Build history of the part. All positions in model axes, mm. A direction names the side the tool comes from. Round coordinates to 2 decimals unless told otherwise and drop trailing zeros. Write each loop counter-clockwise with the first axis right and the second up, starting at its lowest first coordinate (ties: lowest second). Pieces come first, ordered by that corner, then holes.
Item 1: Band-saw the part on A-A, the plane y = 0. Write the cut outline in (x, z), then the cut area to 3 significant figures.
Item 2: Band-saw the part on B-B, the plane x = -12.5. Write the cut outline in (y, z).
Item 3: 3-axis set-ups, long thin cutter, end or side, ignore diameter. For faces 1 (the flat face through (42, -15, 4)), 2 (the flat face through (16, -15, 8)): which of +Z, -Z, +X, -X, +Y, -Y reach the whole face in a straight line?
Item 4: Drop flat-ended pins along their axis: pin 1 Ø1.5 at (y, z) = (-0.5, 3) entering from -X; pin 2 Ø1.5 at (x, z) = (-21.5, 6) entering from -Y; pin 3 Ø4 at (y, z) = (-6.5, 5) entering from -X; pin 4 Ø9.5 at (x, y) = (39.26, -23) entering from +Z. Give the stop position or say it passes through.
Item 5: Mould opens along Y. For faces 3 (the cylindrical face through (49, -33, 4)), 4 (the cylindrical face through (36.26, -22.87, 4.06)), 5 (the flat face through (16, -15, 0)) say: +Y half, -Y half, draft (parallel to the pull), parting line (faces both ways), or undercut.
Item 6: Wall check: probe 1 along Y at (x, z) = (0, 2); probe 2 along Y at (x, z) = (18, 2.25); probe 3 along X at (y, z) = (-8.5, 1.5). Give the ranges that are in metal, low to high.
Item 7: Band-saw the part on C-C, the plane z = 3.75. Write the cut outline in (x, y), then the cut area to 3 significant figures.
Item 8: Band-saw the part on D-D, the plane y = 28.5. Write the cut outline in (x, z), then the cut area to 3 significant figures.
```python
from build123d import *

# Parameters (mm, degrees)
F0_R     = 20
F1_DEPTH = 8
F2_R     = 5
F3_R     = 3
F4_DEPTH = 8


with BuildPart() as f1:
    # F0 (on Top) → F1 (new body)
    with BuildSketch(Plane.XY):
        with BuildLine():
            Line((50, -15), (31.622777, -15))
            ThreePointArc((31.622777, -15), (-18.708287, 29.580399), (0, -35))
            Line((0, -35), (50, -35))
            Line((50, -35), (50, -15))
        make_face()
        Circle(F0_R, mode=Mode.SUBTRACT)
    extrude(amount=F1_DEPTH)

    # F2
    f2_edges = [f1.edges().sort_by_distance(p)[0] for p in [
        (31.622777, -15, 4),
        (50, -15, 4),
        (50, -35, 4),
    ]]
    fillet(f2_edges, radius=F2_R)

    # F3 (on face) → F4 (cut, through all)
    with BuildSketch(Plane.XY.offset(8)):
        with Locations((39.258757, -23)):
            Circle(F3_R)
    extrude(amount=-F4_DEPTH, mode=Mode.SUBTRACT)


solid = f1.part
```
Results:
1. outline: (-35, 0) - (-20, 0) - (-20, 8) - (-35, 8) - close; (20, 0) - (35, 0) - (35, 8) - (20, 8) - close
1. area: 240 mm2
2. outline: (-32.69, 0) - (-15.61, 0) - (-15.61, 8) - (-32.69, 8) - close; (15.61, 0) - (32.69, 0) - (32.69, 8) - (15.61, 8) - close
3. face 1: +Z, -Z, +X, +Y
3. face 2: +Z, +X, -X, +Y, -Y
4. pin 1: stops at x = -35
4. pin 2: stops at y = -28.19
4. pin 3: stops at x = -34.71
4. pin 4: stops at z = 8
5. face 3: -Y half
5. face 4: undercut
5. face 5: draft
6. probe 1: y = -35 to -20, 20 to 35
6. probe 2: y = -35 to -8.72, 8.72 to 30.02
6. probe 3: x = -33.95 to -18.1, 18.1 to 33.95
7. outline: (0, -35) - (45, -35) arc R5 ccw to (50, -30) - (50, -20) arc R5 ccw to (45, -15) - (38.73, -15) arc R5 cw to (33.89, -8.75) arc R35 ccw (long way) to start; hole circle Ø40 at (0, 0); hole circle Ø6 at (39.26, -23)
7. area: 3,110 mm2
8. outline: (-20.32, 0) - (20.32, 0) - (20.32, 8) - (-20.32, 8) - close
8. area: 325 mm2
